```python
from build123d import *

# Parameters (mm, degrees)
F0_W     = 97
F0_H     = 58
F1_DEPTH = 3
F2_W     = 97
F2_H     = 58
F2_W_2   = 92
F2_H_2   = 53
F3_DEPTH = 20
F4_W     = 97
F4_H     = 3
F5_DEPTH = 11
F6_W     = 97
F6_H     = 2.5
F7_DEPTH = 40
F8_W     = 97
F8_H     = 3
F9_DEPTH = 60


with BuildPart() as f1:
    # F0 (on Top) → F1 (new body)
    with BuildSketch(Plane.XY):
        with Locations((48.5, -29)):
            Rectangle(F0_W, F0_H)
    extrude(amount=F1_DEPTH)

    # F2 (on face) → F3 (join)
    with BuildSketch(Plane.XY.offset(3)):
        with Locations((48.5, -29)):
            Rectangle(F2_W, F2_H)
        with Locations((48.5, -29)):
            Rectangle(F2_W_2, F2_H_2, mode=Mode.SUBTRACT)
    extrude(amount=F3_DEPTH)

    # F4 (on face) → F5 (join)
    with BuildSketch(Plane(origin=(0, 0, 0), x_dir=(-1, 0, 0), z_dir=(0, 1, 0))):
        with Locations((-48.5, 1.5)):
            Rectangle(F4_W, F4_H)
    extrude(amount=F5_DEPTH)

    # F6 (on face) → F7 (join)
    with BuildSketch(Plane.XY.offset(23)):
        with Locations((48.5, -1.25)):
            Rectangle(F6_W, F6_H)
    extrude(amount=F7_DEPTH)

    # F8 (on face) → F9 (join, through all)
    with BuildSketch(Plane.XY.offset(3)):
        with Locations((48.5, 9.5)):
            Rectangle(F8_W, F8_H)
    extrude(amount=F9_DEPTH)


solid = f1.part
```
Geometry: final body of the model. Coordinates: model frame, mm. A direction names the side the tool comes from. Coordinates: 2 decimals unless noted, no trailing zeros. Order: outer loops, then holes, each group sorted by start corner. A loop starts at its lowest first (then second) coordinate and runs counter-clockwise, first axis right, second up. Notation, with made-up numbers: (-6.5, 71.5) -> (14.5, 71.5) arc R14 cw to (14.5, 83.5) -> close; hole circle Ø8 at (-21, -9.75). An arc over 180 degrees is marked (long way). Use CSV: the item, a comma, the result in double quotes.
1) Mould query, pull axis X, two halves, no side actions, for faces 1 (the flat face through (48, -29, 3)), 2 (the flat face through (0, -24, 17)), 3 (the flat face through (48, 8, 33)). Classes: +X half, -X half, draft (parallel to the pull), parting line (faces both ways), or undercut.
Findings:
face 1,"undercut"
face 2,"-X half"
face 3,"draft"
2) Section A-A on z = 11.5. Output: boundary loops of the cut face in (x, y), then the cut area to 3 significant figures.
Findings:
outline,"(0, -58) -> (97, -58) -> (97, 0) -> (0, 0) -> close; (0, 8) -> (97, 8) -> (97, 11) -> (0, 11) -> close; hole (2.5, -55.5) -> (94.5, -55.5) -> (94.5, -2.5) -> (2.5, -2.5) -> close"
area,"1,040 mm^2"
3) Access query for faces 4 (the flat face through (48, -57, 23)), 5 (the flat face through (49, 4, 3)), 6 (the flat face through (48, -2.5, 33)). Directions: +Z, -Z, +X, -X, +Y, -Y. A direction counts if a zero-diameter tool reaches every point of the face in a straight line with its end or side. Return the directions, or none.
Findings:
face 4,"+Z, +X, -X, -Y"
face 5,"+Z, +X, -X"
face 6,"+Z"
4) Section B-B on z = 43.5. Output: boundary loops of the cut face in (x, y).
Findings:
outline,"(0, -2.5) -> (97, -2.5) -> (97, 0) -> (0, 0) -> close; (0, 8) -> (97, 8) -> (97, 11) -> (0, 11) -> close"
5) Line query: line 1 (Y direction, x = 20.5, z = 21); line 2 (Y direction, x = 71, z = 32.5); line 3 (X direction, y = -30.5, z = 12). Output: solid intervals per line, ascending.
Findings:
line 1,"y = -58 to -55.5, -2.5 to 0, 8 to 11"
line 2,"y = -2.5 to 0, 8 to 11"
line 3,"x = 0 to 2.5, 94.5 to 97"
6) Section D-D on x = 7. Output: boundary loops of the cut face in (y, z), then the cut area to 3 significant figures.
Findings:
outline,"(-58, 0) -> (11, 0) -> (11, 63) -> (8, 63) -> (8, 3) -> (0, 3) -> (0, 63) -> (-2.5, 63) -> (-2.5, 3) -> (-55.5, 3) -> (-55.5, 23) -> (-58, 23) -> close"
area,"587 mm^2"
7) Section C-C on y = -42. Output: boundary loops of the cut face in (x, z).
Findings:
outline,"(0, 0) -> (97, 0) -> (97, 23) -> (94.5, 23) -> (94.5, 3) -> (2.5, 3) -> (2.5, 23) -> (0, 23) -> close"
8) Pin query (flat end, axial travel): pin 1 Ø2.5 at (x, y) = (27, 6) entering from +Z; pin 2 Ø6 at (x, z) = (81.5, 46.5) entering from -Y. Return the tip coordinate at first contact, or that it passes through.
Findings:
pin 1,"stops at z = 3"
pin 2,"stops at y = -2.5"
